```python
from build123d import *

# Parameters (mm, degrees)
PAD_DEPTH    = 5.2
SKETCH001_R  = 0.4
PAD001_DEPTH = 3
PAD002_DEPTH = 5.6
SKETCH003_R  = 1.25
PAD003_DEPTH = 5.4
FILLET_R     = 1


with BuildPart() as part:
    # Sketch → Pad (new body)
    with BuildSketch(Plane.XY):
        Polygon((-4.15, 4), (4.15, 4), (4.15, -4.6), (3.15, -4.6), (3.15, -5.1), (-3.15, -5.1), (-3.15, -4.6), (-4.15, -4.6), align=None)
    extrude(amount=PAD_DEPTH)

    # Sketch001 → Pad001 (join)
    with BuildSketch(Plane.XY):
        with Locations((-2.54, 0)):
            Circle(SKETCH001_R)
        with Locations((2.54, 0)):
            Circle(SKETCH001_R)
        with Locations((-2.54, -5.08)):
            Circle(SKETCH001_R)
        with Locations((2.54, -5.08)):
            Circle(SKETCH001_R)
        with Locations((0, -5.08)):
            Circle(SKETCH001_R)
    extrude(amount=-PAD001_DEPTH)

    # Sketch002 (on DatumPlane) → Pad002 (join)
    with BuildSketch(Plane(origin=(0, 4, 0), x_dir=(-1, 0, 0), z_dir=(0, 1, 0))):
        with BuildLine():
            ThreePointArc((1.35, 5.279086), (-3, 2.6), (1.35, -0.079086))
            Line((1.35, 5.279086), (1.35, -0.079086))
        make_face()
    extrude(amount=PAD002_DEPTH)

    # Sketch003 (on DatumPlane) → Pad003 (join)
    with BuildSketch(Plane(origin=(0, 9.6, 0), x_dir=(-1, 0, 0), z_dir=(0, 1, 0))):
        with Locations((0, 2.6)):
            Circle(SKETCH003_R)
    extrude(amount=PAD003_DEPTH)

    # Fillet
    fillet_edges = [part.edges().sort_by_distance(p)[0] for p in [
        (1.25, 15, 2.6),
    ]]
    fillet(fillet_edges, radius=FILLET_R)


solid = part.part
```
Here's how the part is built. I have some questions about the finished solid (model axes, mm). A direction names the side the tool comes from. Give positions to 0.01 mm unless a question says otherwise; leave off trailing zeros. Order: outer loops, then holes, each group sorted by start corner. A loop starts at its lowest first (then second) coordinate and runs counter-clockwise, first axis right, second up. Notation, with made-up numbers: M -14,42 L 19,42 A24 ccw 19,78 Z; hole C 47,-30 d10. An arc over 180 degrees is marked long. Use a Markdown table: item, result. Add a question column.
1. I need wall thicknesses on probe 1 along Y at (x, z) = (2, 3.25); probe 2 along Y at (x, z) = (-0.75, 5.25); probe 3 along Z at (x, y) = (3.5, 0.5). Which ranges of each line are inside material? Lowest first, please. Write a range as from..to.
2. For pin 1 Ø2 at (x, z) = (0, 2) entering from +Y; pin 2 Ø2.5 at (x, y) = (0.5, -0.5) entering from -Z; pin 3 Ø2.5 at (y, z) = (8, 3.5) entering from -X; pin 4 Ø2 at (x, y) = (-1.5, 9.5) entering from -Z, each with a flat end and sliding along its axis, tell me the tip position at first contact or that it passes through.
3. On a 3-axis mill with a long thin cutter (end or side, diameter ignored), from which of +Z, -Z, +X, -X, +Y, -Y can I reach the whole of each face in a straight line? I mean faces 5 (the flat face through (0, 0, 5.2)), 6 (the flat face through (3.4, 4, 2.6)), 7 (the cylindrical face through (3, 6.8, 2.7)). Say none if no direction works.
4. Suppose I cut it at D-D (z = 1). List the corners of the cut face in (x, y) for me, and give its area (3 significant figures).
5. Suppose I cut it at A-A (z = -1). List the corners of the cut face in (x, y) for me.
6. Suppose I cut it at B-B (y = 0). List the corners of the cut face in (x, z) for me, and give its area (3 significant figures).
7. If we mould it in two halves opening along X, with no side actions, what happens to faces 1 (the cylindrical face through (-2.16, -4.96, -1.48)), 2 (the cylindrical face through (0.27, 11.77, 1.38)), 3 (the flat face through (-1.35, 7, 3)), 4 (the flat face through (-4, -4.6, 3))? For each: +X half, -X half, draft (parallel to the pull), parting line (faces both ways), or undercut.
8. Suppose I cut it at C-C (x = 2.54). List the corners of the cut face in (y, z) for me.
Results list:
| question | item | result |
|---|---|---|
| 1 | probe 1 | y = -5.1..9.6 |
| 1 | probe 2 | y = 4..9.6 |
| 1 | probe 3 | z = 0..5.2 |
| 2 | pin 1 | stops at y = 15 |
| 2 | pin 2 | stops at z = 0 |
| 2 | pin 3 | stops at x = -1.35 |
| 2 | pin 4 | stops at z = -0.36 |
| 3 | face 5 | +Z, +X, -X, -Y |
| 3 | face 6 | +X, +Y |
| 3 | face 7 | +Y |
| 4 | outline | M -4.15,-4.6 L -3.15,-4.6 L -3.15,-5.1 L 3.15,-5.1 L 3.15,-4.6 L 4.15,-4.6 L 4.15,4 L 2.54,4 L 2.54,9.6 L -1.35,9.6 L -1.35,4 L -4.15,4 Z |
| 4 | area | 96.3 mm² |
| 5 | outline | C -2.54,-5.08 d0.8; C -2.54,0 d0.8; C 0,-5.08 d0.8; C 2.54,-5.08 d0.8; C 2.54,0 d0.8 |
| 6 | outline | M -4.15,0 L -2.94,0 L -2.94,-3 L -2.14,-3 L -2.14,0 L 2.14,0 L 2.14,-3 L 2.94,-3 L 2.94,0 L 4.15,0 L 4.15,5.2 L -4.15,5.2 Z |
| 6 | area | 48.0 mm² |
| 7 | face 1 | undercut |
| 7 | face 2 | parting line |
| 7 | face 3 | -X half |
| 7 | face 4 | draft |
| 8 | outline | M -5.48,-3 L -4.68,-3 L -4.68,0 L -0.4,0 L -0.4,-3 L 0.4,-3 L 0.4,0 L 4,0 L 4,1 L 9.6,1 L 9.6,4.2 L 4,4.2 L 4,5.2 L -5.1,5.2 L -5.1,0 L -5.48,0 Z |
